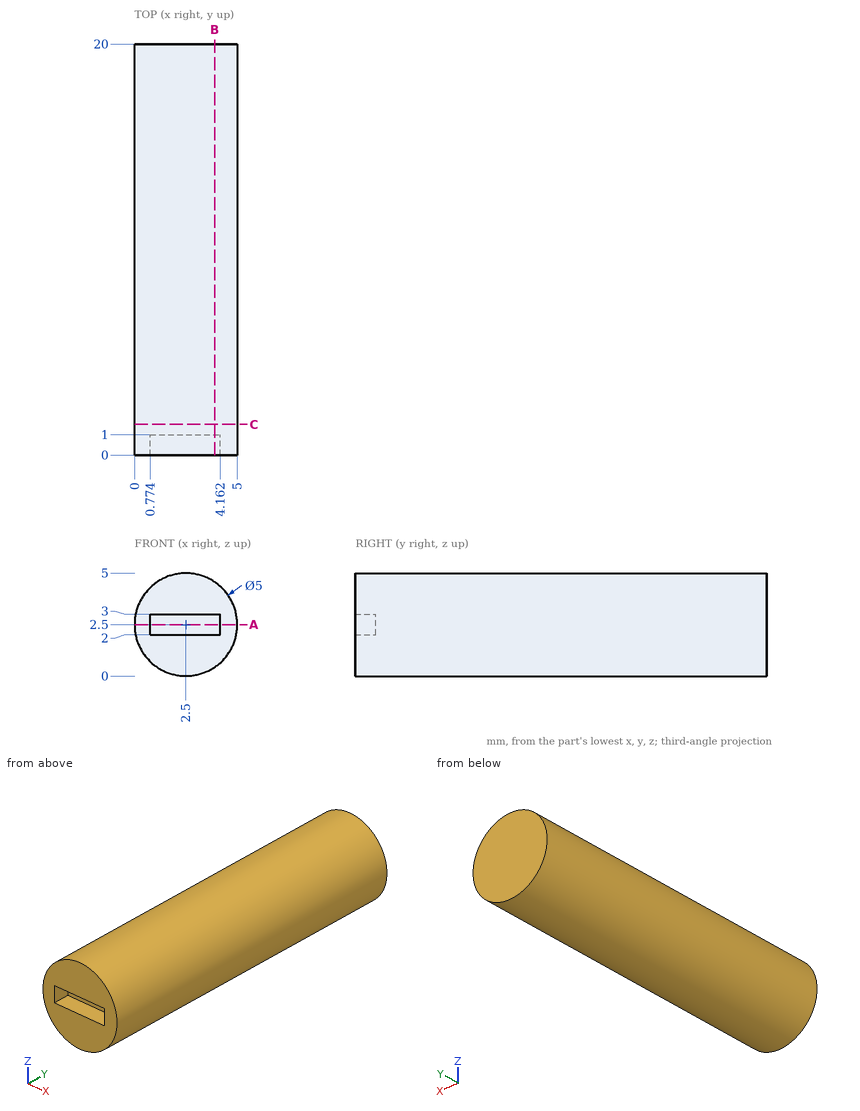
Input: dimensioned drawing with shaded views. Units: mm. Origin: part minimum x, y, z. Coordinates: 2 decimals unless noted, no trailing zeros. Order: outer loops, then holes, each group sorted by start corner. A loop starts at its lowest first (then second) coordinate and runs counter-clockwise, first axis right, second up. Notation, with made-up numbers: (26, 34.25) - (58, 34.25) arc R6 cw to (58, 40.25) - close; hole circle Ø2 at (33, -23). An arc over 180 degrees is marked (long way). Return JSON: item names as keys, results as strings. Group by question number.
1. Pin query (flat end, axial travel): pin 1 (0.8 mm diameter, centred on x = 2, y = 0.5, fed in from +Z). Return the tip coordinate at first contact, or that it passes through.
2. Cut plane A-A (z = 2.5). Output: boundary loops of the cut face in (x, y).
3. Cut plane B-B (x = 3.9). Output: boundary loops of the cut face in (y, z).
4. Material intervals for line 1 along Y through (x, z) = (3.6, 2.3); line 2 along X through (y, z) = (6.5, 3.1); line 3 along X through (y, z) = (16.25, 4.05), sorted ascending. Write a range as [from, to].
5. Cut plane C-C (y = 1.5). Output: boundary loops of the cut face in (x, z), plus the area to 3 significant figures.
Resolved:
{
 "1": {"pin 1": "stops at z = 5"},
 "2": {"outline": "(0, 0) - (0.77, 0) - (0.77, 1) - (4.16, 1) - (4.16, 0) - (5, 0) - (5, 20) - (0, 20) - close"},
 "3": {"outline": "(0, 0.43) - (20, 0.43) - (20, 4.57) - (0, 4.57) - (0, 3) - (1, 3) - (1, 2) - (0, 2) - close"},
 "4": {"line 1": "y = [1, 20]", "line 2": "x = [0.07, 4.93]", "line 3": "x = [0.54, 4.46]"},
 "5": {"outline": "circle Ø5 at (2.5, 2.5)", "area": "19.6 mm²"}
}
